CAD build for the part. Positions are in the model's coordinates, mm. Face numbers are marked on the shaded views. A direction names the side the tool comes from. Give positions to 0.01 mm unless a question says otherwise; leave off trailing zeros. Order: outer loops, then holes, each group sorted by start corner. A loop starts at its lowest first (then second) coordinate and runs counter-clockwise, first axis right, second up.
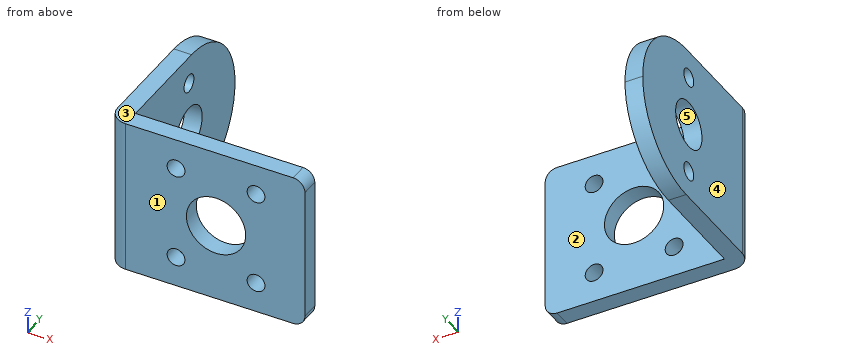
```python
from build123d import *

# Parameters (mm, degrees)
SKETCH1_W               = 30.25
SKETCH1_H               = 26.4
BOSS_EXTRUDE1_DEPTH     = 3
SKETCH1_3_W             = 3
SKETCH1_3_H             = 26.4
BOSS_EXTRUDE2_DEPTH     = 33.25
FILLET1_R               = 3
CUT_EXTRUDE1_DEPTH      = 47.849386335
CUT_EXTRUDE1_DEPTH_BACK = 47.849386335
FILLET2_R               = 2
SKETCH3_R               = 4
SKETCH3_R_2             = 1.5
CUT_EXTRUDE2_DEPTH      = 47.849386335
CUT_EXTRUDE3_REACH      = 38.955
SKETCH4_R               = 5
SKETCH4_R_2             = 1.5


with BuildPart() as part:
    # Sketch1 → Boss-Extrude1 (new body)
    with BuildSketch(Plane(origin=(0, 0, 0), x_dir=(1, 0, 0), z_dir=(0, 1, 0))):
        with Locations((1.5, 0)):
            Rectangle(SKETCH1_W, SKETCH1_H)
    extrude(amount=BOSS_EXTRUDE1_DEPTH)

    # Sketch1<3> → Boss-Extrude2 (add)
    with BuildSketch(Plane(origin=(0, 0, 0), x_dir=(1, 0, 0), z_dir=(0, 1, 0))):
        with Locations((-15.125, 0)):
            Rectangle(SKETCH1_3_W, SKETCH1_3_H)
    extrude(amount=BOSS_EXTRUDE2_DEPTH)

    # Fillet1
    fillet1_edges = [part.edges().sort_by_distance(p)[0] for p in [
        (-16.625, 0, 0),
    ]]
    fillet(fillet1_edges, radius=FILLET1_R)

    # Sketch2 → Cut-Extrude1 (cut, two sides: drawn at the far end of the back side and taken through both)
    with BuildSketch(Plane(origin=(-13.625, 0, 0), x_dir=(0, 0, -1), z_dir=(1, 0, 0)).offset(-CUT_EXTRUDE1_DEPTH_BACK)):
        with BuildLine():
            Line((-13.2, 33.25), (-13.2, 20.05))
            ThreePointArc((-13.2, 20.05), (-9.333809512, 29.383809512), (0, 33.25))
            Line((0, 33.25), (-13.2, 33.25))
        make_face()
        with BuildLine():
            ThreePointArc((0, 33.25), (9.333809512, 29.383809512), (13.2, 20.05))
            Line((13.2, 20.05), (13.2, 33.25))
            Line((13.2, 33.25), (0, 33.25))
        make_face()
    extrude(amount=CUT_EXTRUDE1_DEPTH + CUT_EXTRUDE1_DEPTH_BACK, mode=Mode.SUBTRACT)

    # Fillet2
    fillet2_edges = [part.edges().sort_by_distance(p)[0] for p in [
        (16.625, 1.5, 13.2),
        (16.625, 1.5, -13.2),
    ]]
    fillet(fillet2_edges, radius=FILLET2_R)

    # Sketch3 → Cut-Extrude2 (cut, through all)
    with BuildSketch(Plane(origin=(-13.625, 0, 0), x_dir=(0, 0, -1), z_dir=(1, 0, 0))):
        with Locations((0, 19.25)):
            Circle(SKETCH3_R)
        with Locations((8.5, 19.25)):
            Circle(SKETCH3_R_2)
        with Locations((-8.5, 19.25)):
            Circle(SKETCH3_R_2)
    extrude(amount=-CUT_EXTRUDE2_DEPTH, mode=Mode.SUBTRACT)

    # Sketch4 → Cut-Extrude3 (cut, up to next)
    with BuildSketch(Plane(origin=(0, 3, 0), x_dir=(1, 0, 0), z_dir=(0, 1, 0)), mode=Mode.PRIVATE) as cut_extrude3_sk1:
        with Locations(Location((1.625, 0, 0), (0, 0, 270))):
            Circle(SKETCH4_R)
    cut_extrude3_tool1 = extrude(cut_extrude3_sk1.sketch, amount=-CUT_EXTRUDE3_REACH, mode=Mode.PRIVATE) & part.part
    # Sketch4 → Cut-Extrude3 (cut, up to next)
    with BuildSketch(Plane(origin=(0, 3, 0), x_dir=(1, 0, 0), z_dir=(0, 1, 0)), mode=Mode.PRIVATE) as cut_extrude3_sk2:
        with Locations(Location((-5.125, -8.042853971, 0), (0, 0, 270))):
            Circle(SKETCH4_R_2)
    cut_extrude3_tool2 = extrude(cut_extrude3_sk2.sketch, amount=-CUT_EXTRUDE3_REACH, mode=Mode.PRIVATE) & part.part
    # Sketch4 → Cut-Extrude3 (cut, up to next)
    with BuildSketch(Plane(origin=(0, 3, 0), x_dir=(1, 0, 0), z_dir=(0, 1, 0)), mode=Mode.PRIVATE) as cut_extrude3_sk3:
        with Locations(Location((8.375, 8.042853971, 0), (0, 0, 270))):
            Circle(SKETCH4_R_2)
    cut_extrude3_tool3 = extrude(cut_extrude3_sk3.sketch, amount=-CUT_EXTRUDE3_REACH, mode=Mode.PRIVATE) & part.part
    # Sketch4 → Cut-Extrude3 (cut, up to next)
    with BuildSketch(Plane(origin=(0, 3, 0), x_dir=(1, 0, 0), z_dir=(0, 1, 0)), mode=Mode.PRIVATE) as cut_extrude3_sk4:
        with Locations(Location((8.375, -8.042853971, 0), (0, 0, 270))):
            Circle(SKETCH4_R_2)
    cut_extrude3_tool4 = extrude(cut_extrude3_sk4.sketch, amount=-CUT_EXTRUDE3_REACH, mode=Mode.PRIVATE) & part.part
    # Sketch4 → Cut-Extrude3 (cut, up to next)
    with BuildSketch(Plane(origin=(0, 3, 0), x_dir=(1, 0, 0), z_dir=(0, 1, 0)), mode=Mode.PRIVATE) as cut_extrude3_sk5:
        with Locations(Location((-5.125, 8.042853971, 0), (0, 0, 270))):
            Circle(SKETCH4_R_2)
    cut_extrude3_tool5 = extrude(cut_extrude3_sk5.sketch, amount=-CUT_EXTRUDE3_REACH, mode=Mode.PRIVATE) & part.part
    add(cut_extrude3_tool1.solids().sort_by_distance((1.625, 3, 0))[0], mode=Mode.SUBTRACT)
    add(cut_extrude3_tool2.solids().sort_by_distance((-5.125, 3, 8.042854))[0], mode=Mode.SUBTRACT)
    add(cut_extrude3_tool3.solids().sort_by_distance((8.375, 3, -8.042854))[0], mode=Mode.SUBTRACT)
    add(cut_extrude3_tool4.solids().sort_by_distance((8.375, 3, 8.042854))[0], mode=Mode.SUBTRACT)
    add(cut_extrude3_tool5.solids().sort_by_distance((-5.125, 3, -8.042854))[0], mode=Mode.SUBTRACT)


solid = part.part
```
Item 1: Wall check: L1, parallel to Z at x = -15, y = 19; L2, parallel to Y at x = -6.5, z = -9.5; L3, parallel to X at y = 4.5, z = -2 (3 decimals). Give the ranges that are in metal, low to high.
Item 2: Drop flat-ended pins along their axis: pin 1 Ø3 at (y, z) = (18, -9.5) entering from +X (3 decimals); pin 2 Ø2 at (x, y) = (-11, 6.5) entering from +Z; pin 3 Ø13 at (x, z) = (5, 1) entering from +Y. Give the stop position or say it passes through.
Item 3: Slice it at D-D (x = -11.5). Give the cut face in (y, z).
Item 4: Tool access for the marked faces 1 and 2: list every direction of +Z, -Z, +X, -X, +Y, -Y with a clear straight run to the whole face (end or side of a thin tool).
Item 5: Two-plate mould, pull along Z, no slides. Class the marked faces 3, 4 and 5: released by +Z, released by -Z, zero draft, split by the parting line, or undercut.
Item 6: Slice it at B-B (z = -8.5). Give the cut face in (x, y) (3 decimals), and give its area (3 significant figures).
Item 7: Slice it at C-C (x = 5.5). Give the cut face in (y, z).
Item 8: Slice it at A-A (y = 19.25). Give the cut face in (x, z) (3 decimals), and give its area (3 significant figures).
A:
1. L1: z = -13.2 to -9.98, -7.02 to -3.99, 3.99 to 7.02, 9.98 to 13.2
1. L2: y = 0 to 3
1. L3: x = -16.625 to -13.625
2. pin 1: stops at x = -13.625
2. pin 2: passes through
2. pin 3: stops at y = 3
3. outline: (0, -13.2) - (3, -13.2) - (3, 13.2) - (0, 13.2) - close
4. face 1: +Z, -Z, +X, -X, -Y
4. face 2: +Z, -Z, +X, +Y
5. face 3: released by +Z
5. face 4: zero draft
5. face 5: undercut
6. outline: (-16.625, 3) arc R3 ccw to (-13.625, 0) - (-6.554, 0) - (-6.554, 3) - (-13.625, 3) - (-13.625, 17.75) - (-16.625, 17.75) - close; (-16.625, 20.75) - (-13.625, 20.75) - (-13.625, 30.149) - (-16.625, 30.149) - close; (-3.696, 0) - (6.946, 0) - (6.946, 3) - (-3.696, 3) - close; (9.804, 0) - (16.625, 0) - (16.625, 3) - (9.804, 3) - close
6. area: 153 mm2
7. outline: (0, -13.2) - (3, -13.2) - (3, -3.16) - (0, -3.16) - close; (0, 3.16) - (3, 3.16) - (3, 13.2) - (0, 13.2) - close
8. outline: (-16.625, -13.2) - (-13.625, -13.2) - (-13.625, -10) - (-16.625, -10) - close; (-16.625, -7) - (-13.625, -7) - (-13.625, -4) - (-16.625, -4) - close; (-16.625, 4) - (-13.625, 4) - (-13.625, 7) - (-16.625, 7) - close; (-16.625, 10) - (-13.625, 10) - (-13.625, 13.2) - (-16.625, 13.2) - close
8. area: 37.2 mm2
